from build123d import *

# Parameters (mm, degrees)
F0_R     = 15
F0_R_2   = 10
F1_DEPTH = 25
F2_DEPTH = 50
F3_R     = 2
F4_SIZE  = 3


with BuildPart() as f1:
    # F0 (on Front) → F1 (new body)
    with BuildSketch(Plane.XZ):
        with BuildLine():
            ThreePointArc((6.454945, -29.297332), (23.384272, -18.792973), (30, 0))
            ThreePointArc((30, 0), (23.384272, 18.792973), (6.454945, 29.297332))
            ThreePointArc((6.454945, 29.297332), (-30, 0), (6.454945, -29.297332))
        make_face()
        Circle(F0_R, mode=Mode.SUBTRACT)
        with BuildLine():
            ThreePointArc((6.454945, 29.297332), (23.384272, 18.792973), (30, 0))
            ThreePointArc((30, 0), (23.384272, -18.792973), (6.454945, -29.297332))
            Line((6.454945, -29.297332), (60, -17.5))
            ThreePointArc((60, -17.5), (42.5, 0), (60, 17.5))
            Line((60, 17.5), (6.454945, 29.297332))
        make_face()
        with BuildLine():
            ThreePointArc((77.5, 0), (72.374369, 12.374369), (60, 17.5))
            ThreePointArc((60, 17.5), (42.5, 0), (60, -17.5))
            ThreePointArc((60, -17.5), (72.374369, -12.374369), (77.5, 0))
        make_face()
        with Locations((60, 0)):
            Circle(F0_R_2, mode=Mode.SUBTRACT)
    extrude(amount=F1_DEPTH)

    # F0 (on Front) → F2 (join)
    with BuildSketch(Plane.XZ):
        with BuildLine():
            ThreePointArc((6.454945, -29.297332), (23.384272, -18.792973), (30, 0))
            ThreePointArc((30, 0), (23.384272, 18.792973), (6.454945, 29.297332))
            ThreePointArc((6.454945, 29.297332), (-30, 0), (6.454945, -29.297332))
        make_face()
        Circle(F0_R, mode=Mode.SUBTRACT)
    extrude(amount=F2_DEPTH)

    # F3
    f3_edges = [f1.edges().sort_by_distance(p)[0] for p in [
        (33.227472, 0, -23.398666),
        (-6.454945, -50, 29.297332),
        (77.5, 0, 0),
        (-30, 0, 0),
        (33.227472, 0, 23.398666),
    ]]
    fillet(f3_edges, radius=F3_R)

    # F4
    f4_edges = [f1.edges().sort_by_distance(p)[0] for p in [
        (-15, -50, 0),
        (50, -25, 0),
    ]]
    chamfer(f4_edges, length=F4_SIZE)


solid = f1.part
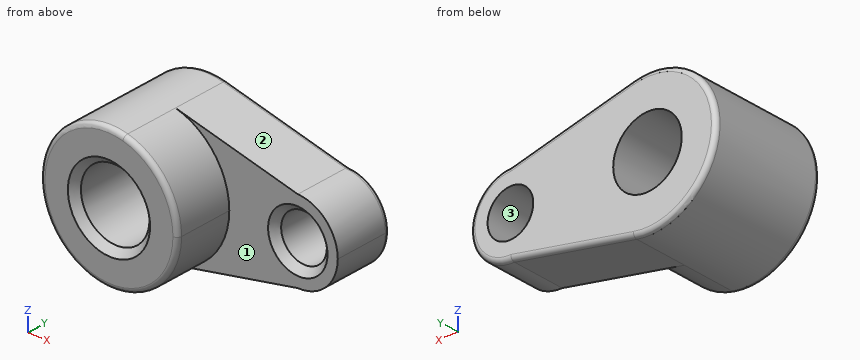
Model file for the job. Use its own axes, mm. Face numbers are marked on the shaded views. Give positions to 0.01 mm unless a question says otherwise; leave off trailing zeros. Loops run counter-clockwise (first coordinate to the right, second up) from the corner with the lowest first, then second, coordinate; pieces in that order, holes last.
1) Saw through at C-C (z = -4). Count the separate pieces of the cut face and the enclosed holes in it, plus the area to 3 significant figures.
2) Saw through at A-A (y = -11). Write the cut outline in (x, z).
3) Wall check: line 1 (Z direction, x = 0, y = -21.5); line 2 (X direction, y = -16, z = 1); line 3 (X direction, y = -21.5, z = 8). Give the ranges that are in metal, low to high.
4) Saw through at B-B (y = -27). Write the cut outline in (x, z).
5) Flat gauge pins, fed straight in: pin 1 Ø1 at (y, z) = (-6.5, 9) entering from +X; pin 2 Ø5 at (x, z) = (36.5, 18.5) entering from -Y; pin 3 Ø18 at (x, z) = (60, 0) entering from +Y; pin 4 Ø12 at (x, y) = (34.5, -12.5) entering from -Z. Where does each tip first touch, or does it go through?
6) Pull direction Z, two halves, no side cores. Call the marked faces 1, 2 and 3: +Z half, -Z half, draft (parallel to the pull), parting line (faces both ways), or undercut.
Answer block:
1. separate pieces: 3
1. enclosed holes: 0
1. area: 2,230 mm2
2. outline: (6.45, -29.3) - (60, -17.5) arc R17.5 ccw to (77.5, 0) arc R17.5 ccw to (60, 17.5) - (6.45, 29.3) arc R30 ccw (long way) to start; hole circle Ø30 at (0, 0); hole circle Ø20 at (60, 0)
3. line 1: z = -30 to -15, 15 to 30
3. line 2: x = -29.98 to -14.97, 14.97 to 50.05, 69.95 to 77.47
3. line 3: x = -28.91 to -12.69, 12.69 to 54, 66 to 75.56
4. outline: (6.45, -29.3) arc R30 ccw to (30, 0) arc R30 ccw to (6.45, 29.3) arc R30 ccw (long way) to start; hole circle Ø30 at (0, 0)
5. pin 1: stops at x = 75.3
5. pin 2: stops at y = -25
5. pin 3: passes through
5. pin 4: stops at z = -24.44
6. face 1: draft
6. face 2: +Z half
6. face 3: undercut
